Job drawing, mm, ordinate dimensions from the low corner. One solid piece. Give positions to 0.01 mm unless a question says otherwise; leave off trailing zeros. Loops run counter-clockwise (first coordinate to the right, second up) from the corner with the lowest first, then second, coordinate; pieces in that order, holes last. Notation, with made-up numbers: M -16.5,47.25 L -12.5,47.25 A30 ccw -12.5,83.25 Z; hole C 67,74 d3. An arc over 180 degrees is marked long. One line per question, with ' | ' between items.
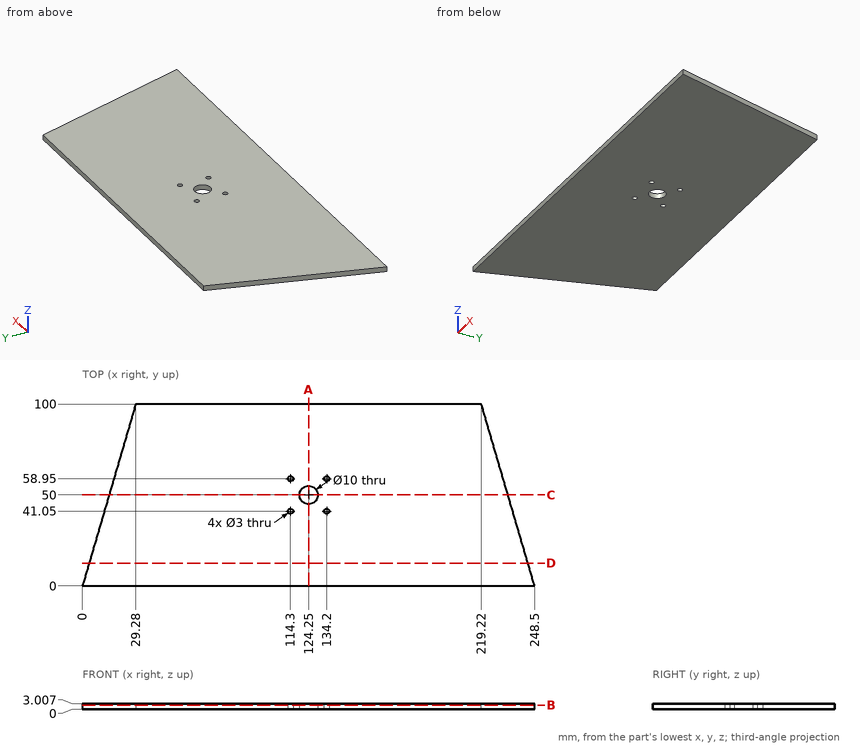
Item 1: Drill centre lines: line 1 along Y through (x, z) = (134.2, 1); line 2 along X through (y, z) = (4, 2.3); line 3 along X through (y, z) = (38, 2.3). Where is each one in solid material? Low to high. Write a range as [from, to].
Conclusion:
line 1: [0, 39.55], [42.55, 57.45], [60.45, 100] | line 2: [1.17, 247.33] | line 3: [11.13, 237.37]
Item 2: Saw through at B-B on z = 2.3. Give the cut face in (x, y), and give its area (3 significant figures).
Conclusion:
outline: M 0,0 L 248.5,0 L 219.22,100 L 29.28,100 Z; hole C 114.3,41.05 d3; hole C 114.3,58.95 d3; hole C 124.25,50 d10; hole C 134.2,41.05 d3; hole C 134.2,58.95 d3 | area: 21,800 mm²
Item 3: Saw through at D-D on y = 12.5. Give the cut face in (x, z), and give its area (3 significant figures).
Conclusion:
outline: M 3.66,0 L 244.84,0 L 244.84,3.01 L 3.66,3.01 Z | area: 725 mm²
Item 4: Saw through at A-A on x = 124.25. Give the cut face in (y, z).
Conclusion:
outline: M 0,0 L 45,0 L 45,3.01 L 0,3.01 Z; M 55,0 L 100,0 L 100,3.01 L 55,3.01 Z
Item 5: Saw through at C-C on y = 50. Give the cut face in (x, z).
Conclusion:
outline: M 14.64,0 L 119.25,0 L 119.25,3.01 L 14.64,3.01 Z; M 129.25,0 L 233.86,0 L 233.86,3.01 L 129.25,3.01 Z
